Autodesk Inventor part; units mm, degrees
ref_plane "YZ Plane" through (0, 0, 0) normal (1, 0, 0) x (0, 1, 0)
ref_plane "XZ Plane" through (0, 0, 0) normal (0, 1, 0) x (-1, 0, 0)
ref_plane "XY Plane" through (0, 0, 0) normal (0, 0, 1) x (1, 0, 0)
sketch "Sketch1" plane through (0, 0, 0) normal (0, 0, 1) x (1, 0, 0)
  line L0 (-2.358, 4.2713) -> (4.842, 4.2713)
  line L1 (4.842, 4.2713) -> (4.842, 2.2713)
  line L2 (4.842, 2.2713) -> (-2.358, 2.2713)
  line L3 (-2.358, 2.2713) -> (-2.358, 4.2713)
  line L4 (-2.358, 4.2713) -> (-7.358, 4.2713)
  line L5 (-7.358, 4.2713) -> (-7.358, -3.7287)
  line L6 (-7.358, -3.7287) -> (-2.358, -3.7287)
  line L7 (-2.358, -3.7287) -> (-2.358, 4.2713)
  line L8 (4.842, 4.2713) -> (9.842, 4.2713)
  line L9 (9.842, 4.2713) -> (9.842, -3.7287)
  line L10 (9.842, -3.7287) -> (4.842, -3.7287)
  line L11 (4.842, -3.7287) -> (4.842, 4.2713)
  point P0 (0, 0)
  point P1 (-2.358, 2.2713)
  point P2 (4.842, 2.2713)
  point P3 (-2.358, 2.2713)
  dimension "d0" = 7.2
  dimension "d1" = 2
  dimension "d2" = 8
  dimension "d3" = 5
  dimension "d4" = 5
extrude "Extrusion1" add sketch "Sketch1" along normal blind 12
sketch "Sketch2" plane through (0, 0, 0) normal (0, 0, -1) x (-1, 0, 0)
  line L0 (2.358, 2.2713) -> (-4.842, 2.2713)
  line L1 (-9.842, 4.2713) -> (7.358, 4.2713)
  line L2 (2.358, 2.2713) -> (-4.842, 2.2713)
  line L3 (-4.842, 2.2713) -> (-4.842, 4.2713)
  line L4 (-4.842, 4.2713) -> (2.358, 4.2713)
  line L5 (2.358, 4.2713) -> (2.358, 2.2713)
  line L6 (-4.842, 2.2713) -> (-4.842, -3.7287)
  point P0 (0, 0)
  point P1 (-4.842, 2.2713)
extrude "Extrusion2" add sketch "Sketch2" along normal blind 1.2
sketch "Sketch3" plane through (0, 0, -1.2) normal (0, 0, -1) x (-1, 0, 0)
  line L0 (-9.842, -3.7287) -> (-9.842, 4.2713)
  line L1 (7.358, 4.2713) -> (7.358, -3.7287)
  line L2 (-9.842, 4.2713) -> (7.358, 4.2713)
  line L3 (7.358, 4.2713) -> (7.358, -3.7287)
  line L4 (7.358, -3.7287) -> (-9.842, -3.7287)
  line L5 (-9.842, -3.7287) -> (-9.842, 4.2713)
  point P0 (0, 0)
extrude "Extrusion3" add sketch "Sketch3" along normal blind 1
sketch "Sketch4" plane through (0, 0, 12) normal (0, 0, 1) x (1, 0, 0)
  line L0 (-7.358, -3.7287) -> (-7.358, 4.2713)
  line L1 (9.842, 4.2713) -> (9.842, -3.7287)
  line L2 (-7.358, 2.2713) -> (9.842, 2.2713)
  line L3 (9.842, 2.2713) -> (9.842, -3.7287)
  line L4 (9.842, -3.7287) -> (-7.358, -3.7287)
  line L5 (-7.358, -3.7287) -> (-7.358, 2.2713)
  line L6 (-2.358, 2.2713) -> (4.842, 2.2713)
  point P0 (0, 0)
extrude "Extrusion4" cut sketch "Sketch4" against normal blind 9
sketch "Sketch5" plane through (0, 0, 3) normal (0, 0, 1) x (1, 0, 0)
  line L0 (9.842, 4.2713) -> (-7.358, 4.2713)
  line L1 (-2.358, 2.2713) -> (-2.358, -3.7287)
  line L2 (4.842, -3.7287) -> (4.842, 2.2713)
  point P0 (0, 0)
  point P1 (-5.358, -1.0287)
  point P2 (7.642, -1.0287)
  dimension "d13" = 5.3
  dimension "d14" = 3
  dimension "d15" = 5.3
  dimension "d16" = 2.8
hole "Hole1" at (-5.358, -1.0287, 3) at (7.642, -1.0287, 3) direction (0, 0, -1) diameter 2 depth 5 tip angle 118
sketch "Sketch6" plane through (0, 0, -1.2) normal (0, 0, 1) x (1, 0, 0)
  line L0 (-2.358, 2.2713) -> (-2.358, -3.7287)
  line L1 (4.842, 2.2713) -> (4.842, -3.7287)
  line L2 (-2.358, 2.2713) -> (4.842, 2.2713)
  line L3 (4.842, 2.2713) -> (4.842, -3.7287)
  line L4 (4.842, -3.7287) -> (-2.358, -3.7287)
  line L5 (-2.358, -3.7287) -> (-2.358, 2.2713)
  point P0 (0, 0)
  point P1 (4.842, 2.2713)
extrude "Extrusion5" cut sketch "Sketch6" against normal blind 2
sketch "Sketch7" plane through (-7.358, 4.2713, 12) normal (0, 1, 0) x (1, 0, 0)
  line L0 (0, 14.2) -> (17.2, 14.2)
  line L1 (17.2, 12) -> (17.2, 0)
  line L2 (0, 14.2) -> (17.2, 14.2)
  line L3 (17.2, 14.2) -> (17.2, 0)
  line L4 (17.2, 0) -> (0, 0)
  line L5 (0, 0) -> (0, 14.2)
  point P0 (7.358, 12)
extrude "Extrusion6" cut sketch "Sketch7" against normal blind 0.2
sketch "Sketch8" plane through (-7.358, 4.0713, 12) normal (0, 1, 0) x (1, 0, 0)
  line L0 (0, 14.2) -> (17.2, 14.2)
  circle A0 centre (8.6, 7.2) radius 3.2
  point P0 (7.358, 12)
  dimension "d31" = 7
  dimension "d32" = 6.4
extrude "Extrusion7" cut sketch "Sketch8" against normal blind 2
sketch "Sketch9" plane through (-7.358, 4.0713, 12) normal (0, 1, 0) x (1, 0, 0)
  line L0 (0, 9) -> (0, 0)
  line L1 (0, 0) -> (17.2, 0)
  line L2 (0, 1.6) -> (5, 1.6)
  line L3 (5, 1.6) -> (5, 0)
  line L4 (5, 0) -> (0, 0)
  line L5 (0, 0) -> (0, 1.6)
  point P0 (7.358, 12)
  dimension "d35" = 1.6
  dimension "d36" = 5
extrude "Extrusion8" cut sketch "Sketch9" against normal blind 2
fillet "Fillet1" radius 1 2 edges at (-4.858, 2.2713, 3) (7.342, 2.2713, 3)
fillet "Fillet2" radius 1 3 edges at (-7.358, 3.1713, 10.4) (9.842, 3.1713, 12) (-2.358, 3.1713, 12)
sketch "Sketch10" plane through (0, 0, -2.2) normal (0, 0, -1) x (-1, 0, 0)
  line L0 (7.358, -3.7287) -> (2.358, -3.7287)
  line L1 (-9.842, 4.0713) -> (-9.842, -3.7287)
  line L2 (7.358, -3.7287) -> (-9.842, -3.7287)
  line L3 (-9.842, -3.7287) -> (-9.842, -2.7287)
  line L4 (-9.842, -2.7287) -> (7.358, -2.7287)
  line L5 (7.358, -2.7287) -> (7.358, -3.7287)
  point P0 (0, 0)
  point P1 (-9.842, -3.7287)
  point P2 (2.358, -3.7287)
  dimension "d45" = 1
extrude "Extrusion9" cut sketch "Sketch10" against normal blind 1
fillet "Fillet4" radius 1 2 edges at (-7.358, -3.7287, 1.5) (9.842, -3.7287, 1.5)
chamfer "Chamfer3" distance 1 angle 45 2 edges at (-2.358, -2.7287, -1.7) (4.842, -2.7287, -1.7)
sketch "Sketch11" plane through (0, 0, -2.2) normal (0, 0, -1) x (-1, 0, 0)
  line L0 (-9.842, 2.2713) -> (-4.842, 2.2713)
  line L1 (-5.342, 2.2713) -> (2.858, 2.2713)
  line L2 (2.858, 2.2713) -> (2.858, -3.7287)
  line L3 (2.858, -3.7287) -> (-5.342, -3.7287)
  line L4 (-5.342, -3.7287) -> (-5.342, 2.2713)
  line L5 (-4.842, -1.7287) -> (-4.842, 2.2713)
  line L6 (2.358, 2.2713) -> (2.358, -1.7287)
  line L7 (-4.842, -3.7287) -> (-8.842, -3.7287)
  point P0 (0, 0)
  dimension "d52" = 8.2
  dimension "d53" = 0.5
  dimension "d54" = 0.5
extrude "Extrusion10" cut sketch "Sketch11" against normal blind 10
sketch "Sketch12" plane through (-7.358, 4.0713, 12) normal (0, 1, 0) x (1, 0, 0)
  line L0 (0, 2.6) -> (0, 12)
  line L1 (1, 1.6) -> (5, 1.6)
  point P0 (7.358, 12)
  point P1 (2.1, 4)
  dimension "d57" = 2.1
  dimension "d58" = 2.4
hole "Hole2" at (-5.258, 4.0713, 8) direction (0, -1, 0) diameter 2 depth 5 tip angle 118 countersink diameter 4 countersink angle 90
properties part number "switch-mount"
The listing builds one solid part. Answer for the finished solid, in the listing's coordinates (mm). A direction names the side the tool comes from. Coordinates: 2 decimals unless noted, no trailing zeros. Write each loop counter-clockwise with the first axis right and the second up, starting at its lowest first coordinate (ties: lowest second). Pieces come first, ordered by that corner, then holes. Notation, with made-up numbers: (36, -36) - (52, -36) arc R23 ccw to (52, 3) - close; hole circle Ø10 at (-32, 53). An arc over 180 degrees is marked (long way). Answer as CSV lines item,"result".
1. Find section C-C (y = 1). Give the vertices of the cut face in (x, z).
Computed values:
outline,"(-7.36, -2.2) - (-2.86, -2.2) - (-2.86, -1.2) - (-7.36, -1.2) - close; (-7.36, 0) - (-2.86, 0) - (-2.86, 3) - (-7.36, 3) - close; (5.34, -2.2) - (9.84, -2.2) - (9.84, -1.2) - (5.34, -1.2) - close; (5.34, 0) - (9.84, 0) - (9.84, 3) - (5.34, 3) - close"
2. Find section A-A (z = 4.8). Give the vertices of the cut face in (x, y), plus the area to 3 significant figures.
Computed values:
outline,"(-7.36, 2.27) - (-1.96, 2.27) - (-1.96, 4.07) - (-7.36, 4.07) - close; (4.44, 2.27) - (9.84, 2.27) - (9.84, 4.07) - (4.44, 4.07) - close"
area,"19.4 mm²"
3. Straight lines are drawn through the part: line 1 (Z direction, x = 9, y = -2.5); line 2 (X direction, y = -0.5, z = 2.25); line 3 (X direction, y = 1, z = 0.5). For each, find the intervals that lie inside material, in ascending order. Write a range as [from, to].
Computed values:
line 1,"z = [-2.2, -1.2], [0, 3]"
line 2,"x = [-7.36, -6.21], [-4.51, -2.86], [5.34, 6.79], [8.49, 9.84]"
line 3,"x = [-7.36, -2.86], [5.34, 9.84]"
4. A tool of negligible diameter and unlimited length cuts with its end or side. For faces 5 (the cylindrical face through (-5.66, -1.98, -1.61)), 6 (the flat face through (5.342, -1, 2)), 7 (the flat face through (4.842, 3, -1)), 8 (the flat face through (-4.9, 0.2, 0)), 9 (the flat face through (1.1, 2.271, 8.2)), from which of +Z, -Z, +X, -X, +Y, -Y can it reach the whole face along a straight path? Write none if from no direction.
Computed values:
face 5,"+Z"
face 6,"+Z, -Z, -Y"
face 7,"+X, +Y, -Y"
face 8,"-X, +Y, -Y"
face 9,"+Z, -Y"
5. Given P1, Ø4, axis at x = 6, z = 5.5, coming from the -Y side; P2, Ø7, axis at x = 0.5, z = 7, coming from the -Y side; P3, Ø1.3, axis at x = -5.5, y = -1.5, coming from the +Z side, each flat-ended and moving along its own axis, determine where each tip first touches the part or whether it passes through.
Computed values:
P1,"stops at y = 2.14"
P2,"stops at y = 2.27"
P3,"stops at z = 3"
6. Find section D-D (x = 1). Give the vertices of the cut face in (y, z).
Computed values:
outline,"(2.27, -2.2) - (4.07, -2.2) - (4.07, 1.61) - (2.27, 1.61) - close; (2.27, 7.99) - (4.07, 7.99) - (4.07, 12) - (2.27, 12) - close"
7. Determine the mould class of faces 1 (the cylindrical face through (9.541, -3.444, 1.521)), 2 (the cylindrical face through (4.198, 3.184, 6.026)), 3 (the flat face through (-5, -3.729, 1)), 4 (the cylindrical face through (-7.06, 3.16, 10.11)) for opening direction X: +X half, -X half, draft (parallel to the pull), parting line (faces both ways), or undercut.
Computed values:
face 1,"+X half"
face 2,"undercut"
face 3,"draft"
face 4,"-X half"
8. Find section B-B (z = 2). Give the vertices of the cut face in (x, y), plus the area to 3 significant figures.
Computed values:
outline,"(-7.36, -2.73) arc R1 ccw to (-6.36, -3.73) - (-2.86, -3.73) - (-2.86, 2.27) - (-0.31, 2.27) - (-0.31, 4.07) - (-7.36, 4.07) - close; (2.79, 2.27) - (5.34, 2.27) - (5.34, -3.73) - (8.84, -3.73) arc R1 ccw to (9.84, -2.73) - (9.84, 4.07) - (2.79, 4.07) - close; hole circle Ø2 at (-5.36, -1.03); hole circle Ø2 at (7.64, -1.03)"
area,"72.7 mm²"
